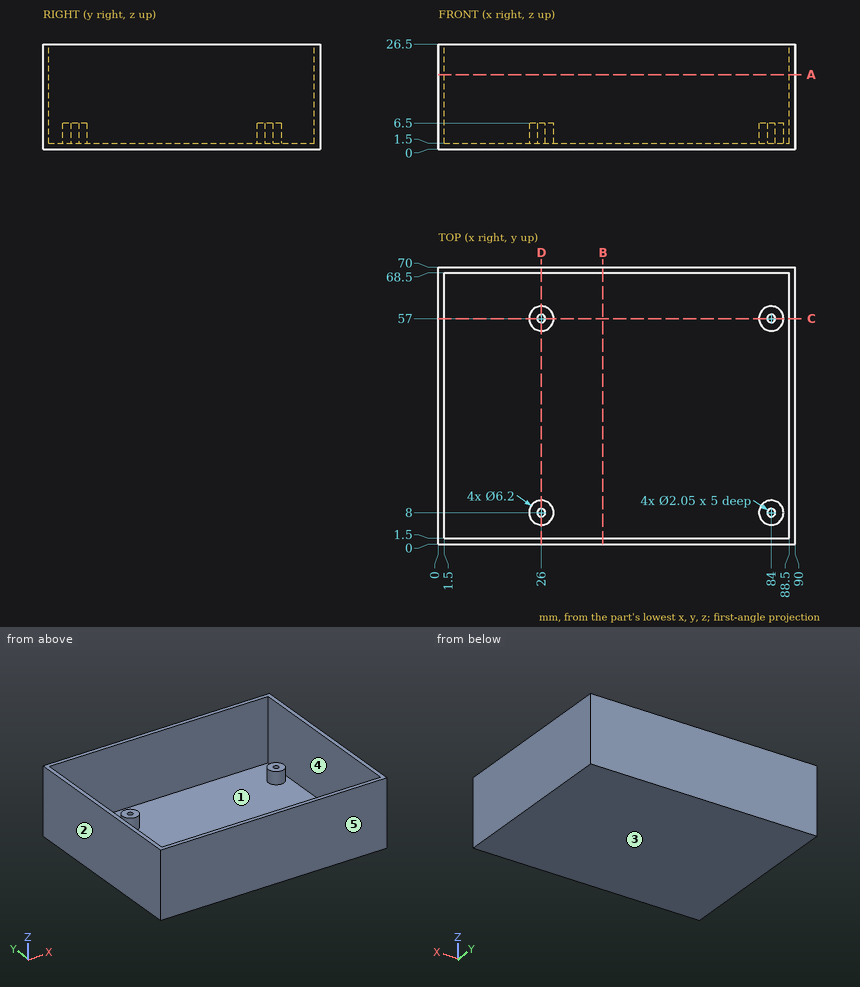
Design review of the part shown in the three views and the two pictorial views. Dimensions are in mm from the part's minimum x, y and z. A direction names the side the tool comes from. Round coordinates to 2 decimals unless told otherwise and drop trailing zeros. Write each loop counter-clockwise with the first axis right and the second up, starting at its lowest first coordinate (ties: lowest second). Pieces come first, ordered by that corner, then holes.
1) For line 1 along Y through (x, z) = (26, 4.4) (3 decimals); line 2 along X through (y, z) = (16, 24); line 3 along Y through (x, z) = (29.5, 5), list the stretches that pass through material, from the lowest coordinate up.
Answer below:
line 1: y = 0 to 1.5, 4.9 to 6.975, 9.025 to 11.1, 53.9 to 55.975, 58.025 to 60.1, 68.5 to 70
line 2: x = 0 to 1.5, 88.5 to 90
line 3: y = 0 to 1.5, 68.5 to 70
2) Machinability: for the marked faces 4 and 5, which of the approach directions +Z, -Z, +X, -X, +Y, -Y give a long, thin tool a straight path to every point of the face, cutting with its end or side? Answer none if there is none.
Answer below:
face 4: +Z
face 5: +Z, -Z, +X, -X, -Y
3) Insertion check: pin 1 Ø1.5 at (x, y) = (70.5, 22) entering from +Z; pin 2 Ø1.9 at (x, y) = (26.5, 57.5) entering from +Z. Each pin has a flat end and moves straight along its axis. Give the tip position at first contact, or say it passes through.
Answer below:
pin 1: stops at z = 1.5
pin 2: stops at z = 6.5
4) Take a section at C-C on y = 57. Give the boundary of the cut face in (x, z) (3 decimals).
Answer below:
outline: (0, 0) - (90, 0) - (90, 26.5) - (88.5, 26.5) - (88.5, 1.5) - (87.1, 1.5) - (87.1, 6.5) - (85.025, 6.5) - (85.025, 1.5) - (82.975, 1.5) - (82.975, 6.5) - (80.9, 6.5) - (80.9, 1.5) - (29.1, 1.5) - (29.1, 6.5) - (27.025, 6.5) - (27.025, 1.5) - (24.975, 1.5) - (24.975, 6.5) - (22.9, 6.5) - (22.9, 1.5) - (1.5, 1.5) - (1.5, 26.5) - (0, 26.5) - close
5) Take a section at B-B on x = 41.5. Give the boundary of the cut face in (y, z).
Answer below:
outline: (0, 0) - (70, 0) - (70, 26.5) - (68.5, 26.5) - (68.5, 1.5) - (1.5, 1.5) - (1.5, 26.5) - (0, 26.5) - close
6) Take a section at A-A on z = 18.75. Give the boundary of the cut face in (x, y).
Answer below:
outline: (0, 0) - (90, 0) - (90, 70) - (0, 70) - close; hole (1.5, 1.5) - (88.5, 1.5) - (88.5, 68.5) - (1.5, 68.5) - close
7) Mouldability with a two-part tool opening along X and no side actions: class the marked faces 1, 2 and 3 as +X half, -X half, draft (parallel to the pull), parting line (faces both ways), or undercut.
Answer below:
face 1: undercut
face 2: -X half
face 3: draft
8) Take a section at D-D on x = 26. Give the boundary of the cut face in (y, z) (3 decimals), then the cut area to 4 significant figures.
Answer below:
outline: (0, 0) - (70, 0) - (70, 26.5) - (68.5, 26.5) - (68.5, 1.5) - (60.1, 1.5) - (60.1, 6.5) - (58.025, 6.5) - (58.025, 1.5) - (55.975, 1.5) - (55.975, 6.5) - (53.9, 6.5) - (53.9, 1.5) - (11.1, 1.5) - (11.1, 6.5) - (9.025, 6.5) - (9.025, 1.5) - (6.975, 1.5) - (6.975, 6.5) - (4.9, 6.5) - (4.9, 1.5) - (1.5, 1.5) - (1.5, 26.5) - (0, 26.5) - close
area: 221.5 mm2
